The listing builds one solid part. Answer for the finished solid, in the listing's coordinates (mm). A direction names the side the tool comes from. Coordinates: 2 decimals unless noted, no trailing zeros. Loops run counter-clockwise (first coordinate to the right, second up) from the corner with the lowest first, then second, coordinate; pieces in that order, holes last. Notation, with made-up numbers: M 51,52 L 75,52 A12 cw 75,71 Z; hole C 89,-5 d1. An arc over 180 degrees is marked long. Return JSON: item names as keys, results as strings. Group by question number.
1. Section C-C (y = 13.5) is taken. Write down the section's boundary in (x, z), then the cut area to 3 significant figures.
2. Given P1, Ø5, axis at y = 15, z = 31.5, coming from the -X side; P2, Ø1, axis at y = 27.5, z = -7, coming from the -X side; P3, Ø4.5, axis at x = 50.5, y = 22.5, coming from the +Z side; P4, Ø3.5, axis at x = 78.5, z = 3, coming from the -Y side, each flat-ended and moving along its own axis, determine where each tip first touches the part or whether it passes through.
3. Section D-D (x = 103.5) is taken. Write down the section's boundary in (y, z), then the cut area to 3 significant figures.
4. Which of the six approach directions +Z, -Z, +X, -X, +Y, -Y give full straight-line access (tool end or side, diameter ignored) to faces 1 (the face through (76, 22, 6)), 2 (the face through (9.86, 9.76, 31)), 3 (the face through (112.745, 39.923, 20.765))?
5. Straight lines are drawn through the part: L1, parallel to Y at x = 8, z = 0; L2, parallel to Z at x = 92, y = 0; L3, parallel to Z at x = 54.5, y = 4. For each, find the intervals that lie inside material, in ascending order. Write a range as from..to.
6. Section A-A (x = 26) is taken. Write down the section's boundary in (y, z).
7. Section B-B (z = 0) is taken. Write down the section's boundary in (x, y), then the cut area to 3 significant figures.
8. The mould has two halves that part along Y. Classify faces 4 (the face through (74.23, -20.983, 0.838)), 5 (the face through (46.84, 15.02, -47.69)), 6 (the face through (0, -33, 1)), 7 (the face through (76, 22, -6)): pulls with the +Y half, pulls with the -Y half, needs draft (parallel to the pull), parting line crosses it, or undercut.
```python
from build123d import *

# Parameters (mm, degrees)
SKETCH1_R                       = 50
SKETCH1_R_2                     = 21
BOSS_EXTRUDE1_DEPTH             = 130
CUT_EXTRUDE1_DEPTH              = 148.986485869
CUT_EXTRUDE1_DEPTH_BACK         = 148.986485869
SKETCH2_W                       = 12
SKETCH2_H                       = 6.6
SKETCH3_W                       = 35
SKETCH3_H                       = 5
SKETCH4_R                       = 32.5
CUT_EXTRUDE2_DEPTH              = 20
M8X1_0_TAPPED_HOLE1_D           = 7
M8X1_0_TAPPED_HOLE1_DEPTH       = 40
M8X1_0_TAPPED_HOLE1_CSINK_D     = 8.05
M8X1_0_TAPPED_HOLE1_CSINK_ANGLE = 90
M8X1_0_TAPPED_HOLE1_TIP         = 2.103012167


with BuildPart() as part:
    # Sketch1 → Boss-Extrude1 (new body)
    with BuildSketch(Plane(origin=(0, 0, 0), x_dir=(0, 0, -1), z_dir=(1, 0, 0))):
        Circle(SKETCH1_R)
        Circle(SKETCH1_R_2, mode=Mode.SUBTRACT)
    extrude(amount=BOSS_EXTRUDE1_DEPTH)

    # Sketch2 → Cut-Extrude1 (cut, two sides: drawn at the far end of the back side and taken through both)
    with BuildSketch(Plane.ZY.offset(-CUT_EXTRUDE1_DEPTH_BACK)):
        with Locations((0, 21)):
            Rectangle(SKETCH2_W, SKETCH2_H)
    extrude(amount=CUT_EXTRUDE1_DEPTH + CUT_EXTRUDE1_DEPTH_BACK, mode=Mode.SUBTRACT)

    # Sketch3 → Cut-Revolve1 (revolve, cut)
    with BuildSketch(Plane(origin=(0, 0, 0), x_dir=(1, 0, 0), z_dir=(0, 1, 0))):
        with Locations((112.5, -47.5)):
            Rectangle(SKETCH3_W, SKETCH3_H)
    revolve(axis=Axis((0, 0, 0), (1, 0, 0)), mode=Mode.SUBTRACT)

    # Sketch4 → Cut-Extrude2 (cut)
    with BuildSketch(Plane.ZY):
        Circle(SKETCH4_R)
    extrude(amount=-CUT_EXTRUDE2_DEPTH, mode=Mode.SUBTRACT)

    # M8x1.0 Tapped Hole1
    with Locations(Plane(origin=(0, 0, -42.5), x_dir=(0, 0, -1), z_dir=(-1, 0, 0))):
        with Locations((0, 0), (-85, 0)):
            CounterSinkHole(M8X1_0_TAPPED_HOLE1_D / 2, M8X1_0_TAPPED_HOLE1_CSINK_D / 2, depth=M8X1_0_TAPPED_HOLE1_DEPTH, counter_sink_angle=M8X1_0_TAPPED_HOLE1_CSINK_ANGLE)
            with Locations((0, 0, -(M8X1_0_TAPPED_HOLE1_DEPTH + M8X1_0_TAPPED_HOLE1_TIP / 2))):  # 118° drill point
                Cone(0, M8X1_0_TAPPED_HOLE1_D / 2, M8X1_0_TAPPED_HOLE1_TIP, mode=Mode.SUBTRACT)


solid = part.part
```
Worked out:
{
 "1": {"outline": "M 0,-48.14 L 95,-48.14 L 95,-42.93 L 130,-42.93 L 130,-16.09 L 20,-16.09 L 20,-29.56 L 0,-29.56 Z; M 0,29.56 L 20,29.56 L 20,16.09 L 130,16.09 L 130,42.93 L 95,42.93 L 95,48.14 L 0,48.14 Z", "area": "7,430 mm^2"},
 "2": {"P1": "x = 0", "P2": "x = 20", "P3": "z = 45.72", "P4": "y = -49.98"},
 "3": {"outline": "C 0,0 d90; hole M 20.12,-6 L 24.3,-6 L 24.3,6 L 20.12,6 A21 ccw long Z", "area": "4,930 mm^2"},
 "4": {"face 1": "+X, -X", "face 2": "-X", "face 3": "+X"},
 "5": {"L1": "-50..-32.5, 32.5..50", "L2": "-50..-21, 21..50", "L3": "-49.84..-20.62, 20.62..49.84"},
 "6": {"outline": "C 0,0 d100; hole C 0,-42.5 d7; hole C 0,42.5 d7; hole M 20.12,-6 L 24.3,-6 L 24.3,6 L 20.12,6 A21 ccw long Z"},
 "7": {"outline": "M 0,-50 L 95,-50 L 95,-45 L 130,-45 L 130,-21 L 20,-21 L 20,-32.5 L 0,-32.5 Z; M 0,32.5 L 20,32.5 L 20,24.3 L 130,24.3 L 130,45 L 95,45 L 95,50 L 0,50 Z", "area": "6,370 mm^2"},
 "8": {"face 4": "undercut", "face 5": "parting line crosses it", "face 6": "needs draft", "face 7": "undercut"}
}
